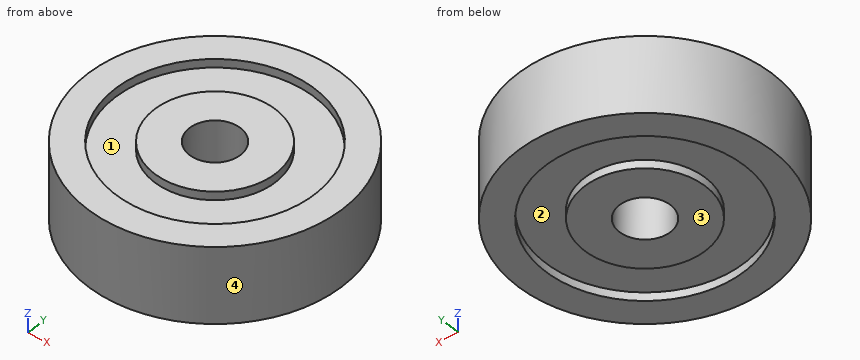
```python
from build123d import *

# Parameters (mm, degrees)
SKETCH_1_R          = 15
SKETCH_1_R_2        = 3
EXTRUDE_1_DEPTH     = 9
SKETCH_2_R          = 11.723129436
SKETCH_2_R_2        = 7.131561965
CUT_EXTRUDE_1_DEPTH = 1


with BuildPart() as part:
    # 草图1 → 凸台-拉伸1 (new body)
    with BuildSketch(Plane.XY):
        Circle(SKETCH_1_R)
        Circle(SKETCH_1_R_2, mode=Mode.SUBTRACT)
    extrude(amount=EXTRUDE_1_DEPTH)

    # 草图2 → 切除-拉伸1 (cut)
    with BuildSketch(Plane(origin=(0, 0, 0), x_dir=(-1, 0, 0), z_dir=(0, 0, -1))):
        Circle(SKETCH_2_R)
        Circle(SKETCH_2_R_2, mode=Mode.SUBTRACT)
    cut_extrude_1 = extrude(amount=-CUT_EXTRUDE_1_DEPTH, mode=Mode.SUBTRACT)

    # 镜向1: 切除-拉伸1 across plane
    add(cut_extrude_1.mirror(Plane(origin=(0, 0, 4.5), x_dir=(1, 0, 0), z_dir=(0, 0, -1))), mode=Mode.SUBTRACT)


solid = part.part
```
For this review, take the finished solid that the model builds, in its own axes (mm). Face numbers are marked on the shaded views. Coordinates: 2 decimals unless noted, no trailing zeros. Loops run counter-clockwise (first coordinate to the right, second up) from the corner with the lowest first, then second, coordinate; pieces in that order, holes last.
1. For line 1 (Y direction, x = 0, z = 8.75); line 2 (Y direction, x = 0, z = 6.5); line 3 (X direction, y = 5, z = 0.75), list the stretches that pass through material, from the lowest coordinate up.
2. Add section D-D, the plane y = -4. Give the boundary of the cut face in (x, z).
3. Add section C-C, the plane z = 4.5. Give the boundary of the cut face in (x, y), then the cut area to 3 significant figures.
4. Mouldability with a two-part tool opening along Y and no side actions: class the marked faces 1, 2, 3 and 4 as +Y half, -Y half, draft (parallel to the pull), parting line (faces both ways), or undercut.
5. Insertion check: P1, Ø5, axis at x = 7.5, z = 8, coming from the +Y side; P2, Ø4, axis at x = -6, z = 5.5, coming from the +Y side; P3, Ø4, axis at x = -11.5, z = 1.5, coming from the +Y side. Each pin has a flat end and moves straight along its axis. Give the tip position at first contact, or say it passes through.
6. Add section A-A, the plane x = 0. Give the boundary of the cut face in (y, z).
Result:
1. line 1: y = -15 to -11.72, -7.13 to -3, 3 to 7.13, 11.72 to 15
1. line 2: y = -15 to -3, 3 to 15
1. line 3: x = -14.14 to -10.6, -5.09 to 5.09, 10.6 to 14.14
2. outline: (-14.46, 0) - (-11.02, 0) - (-11.02, 1) - (-5.9, 1) - (-5.9, 0) - (5.9, 0) - (5.9, 1) - (11.02, 1) - (11.02, 0) - (14.46, 0) - (14.46, 9) - (11.02, 9) - (11.02, 8) - (5.9, 8) - (5.9, 9) - (-5.9, 9) - (-5.9, 8) - (-11.02, 8) - (-11.02, 9) - (-14.46, 9) - close
3. outline: circle Ø30 at (0, 0); hole circle Ø6 at (0, 0)
3. area: 679 mm2
4. face 1: undercut
4. face 2: undercut
4. face 3: draft
4. face 4: parting line
5. P1: stops at y = 14.14
5. P2: stops at y = 14.46
5. P3: stops at y = 11.61
6. outline: (-15, 0) - (-11.72, 0) - (-11.72, 1) - (-7.13, 1) - (-7.13, 0) - (-3, 0) - (-3, 9) - (-7.13, 9) - (-7.13, 8) - (-11.72, 8) - (-11.72, 9) - (-15, 9) - close; (3, 0) - (7.13, 0) - (7.13, 1) - (11.72, 1) - (11.72, 0) - (15, 0) - (15, 9) - (11.72, 9) - (11.72, 8) - (7.13, 8) - (7.13, 9) - (3, 9) - close
